Input: part model. Units: mm. Frame: model coordinates. A direction names the side the tool comes from. Round coordinates to 2 decimals unless told otherwise and drop trailing zeros. Loops run counter-clockwise (first coordinate to the right, second up) from the corner with the lowest first, then second, coordinate; pieces in that order, holes last. Notation, with made-up numbers: (38.25, 15) - (46.25, 15) arc R16 ccw to (46.25, 23) - close; hole circle Ø2 at (30.25, -35.75). An arc over 180 degrees is marked (long way). Write each question's results on one line, items separated by ' | '.
from build123d import *

# Parameters (mm, degrees)
BOSS_EXTRUDE1_DEPTH = 20
BOSS_EXTRUDE5_DEPTH = 5
SKETCH12_R          = 3
CUT_EXTRUDE7_DEPTH  = 88.776628115
SKETCH13_R          = 3
CUT_EXTRUDE8_DEPTH  = 87.566562518
SKETCH14_R          = 3
CUT_EXTRUDE9_DEPTH  = 91.441895398


with BuildPart() as part:
    # Sketch1 → Boss-Extrude1 (new body)
    with BuildSketch(Plane(origin=(0, 0, 0), x_dir=(1, 0, 0), z_dir=(0, 1, 0))):
        Polygon((0, 50), (0, 0), (40, 0), (40, 5), (5, 5), (5, 50), align=None)
    extrude(amount=BOSS_EXTRUDE1_DEPTH)

    # Sketch11 → Boss-Extrude5 (add)
    with BuildSketch(Plane(origin=(0, 20, 0), x_dir=(1, 0, 0), z_dir=(0, 1, 0))):
        Polygon((0, 0), (0, 15), (61.191009328, 48.995005183), (71.096669706, 31.164816504), (15, 0), align=None)
    extrude(amount=BOSS_EXTRUDE5_DEPTH)

    # Sketch12 → Cut-Extrude7 (cut, through all)
    with BuildSketch(Plane(origin=(0, 0, -5), x_dir=(-1, 0, 0), z_dir=(0, 0, -1))):
        with Locations((-10, 10)):
            Circle(SKETCH12_R)
        with Locations((-30, 10)):
            Circle(SKETCH12_R)
    extrude(amount=-CUT_EXTRUDE7_DEPTH, mode=Mode.SUBTRACT)

    # Sketch13 → Cut-Extrude8 (cut, through all)
    with BuildSketch(Plane(origin=(5, 0, 0), x_dir=(0, 0, -1), z_dir=(1, 0, 0))):
        with Locations((15, 10)):
            Circle(SKETCH13_R)
        with Locations((35, 10)):
            Circle(SKETCH13_R)
    extrude(amount=-CUT_EXTRUDE8_DEPTH, mode=Mode.SUBTRACT)

    # Sketch14 → Cut-Extrude9 (cut, through all)
    with BuildSketch(Plane(origin=(0, 25, 0), x_dir=(1, 0, 0), z_dir=(0, 1, 0))):
        with Locations(Location((57.323641314, 35.365007327, 0), (0, 0, 270))):
            Circle(SKETCH14_R)
        with Locations(Location((39.685556362, 25.936435896, 0), (0, 0, 270))):
            Circle(SKETCH14_R)
    extrude(amount=-CUT_EXTRUDE9_DEPTH, mode=Mode.SUBTRACT)


solid = part.part
1. Section query B-B, the plane y = 10. Output: boundary loops of the cut face in (x, z), plus the area to 3 significant figures.
Answer:
outline: (0, -50) - (5, -50) - (5, -38) - (0, -38) - close; (0, -32) - (5, -32) - (5, -18) - (0, -18) - close; (0, -12) - (5, -12) - (5, -5) - (7, -5) - (7, 0) - (0, 0) - close; (13, -5) - (27, -5) - (27, 0) - (13, 0) - close; (33, -5) - (40, -5) - (40, 0) - (33, 0) - close | area: 305 mm^2
2. Line query: line 1 (Y direction, x = 30, z = -2.2); line 2 (X direction, y = 3, z = -30.5); line 3 (Y direction, x = 2, z = -15). Output: solid intervals per line, ascending. Write a range as [from, to].
Answer:
line 1: [0, 7], [13, 20] | line 2: [0, 5] | line 3: [0, 7], [13, 25]
3. Section query D-D, the plane x = 10. Output: boundary loops of the cut face in (y, z), plus the area to 3 significant figures.
Answer:
outline: (0, -5) - (7, -5) - (7, 0) - (0, 0) - close; (13, -5) - (20, -5) - (20, -20.56) - (25, -20.56) - (25, 0) - (13, 0) - close | area: 173 mm^2
4. Section query A-A, the plane z = -30. Output: boundary loops of the cut face in (x, y), plus the area to 3 significant figures.
Answer:
outline: (0, 0) - (5, 0) - (5, 20) - (0, 20) - close; (27, 20) - (69, 20) - (69, 25) - (27, 25) - close | area: 310 mm^2
5. Contact query for flat-ended pins moving along their axis: pin 1 (4 mm diameter, centred on y = 5.5, z = -43.5, fed in from +X); pin 2 (2.5 mm diameter, centred on x = 1.5, z = -25, fed in from +Y); pin 3 (12 mm diameter, centred on x = 34, y = 22.5, fed in from +Z); pin 4 (12 mm diameter, centred on x = 59.5, y = 13, fed in from +Z). Output: stop coordinate, or through.
Answer:
pin 1: x = 5 | pin 2: y = 20 | pin 3: z = 0 | pin 4: through
6. Section query C-C, the plane z = -3. Output: boundary loops of the cut face in (x, y), plus the area to 3 significant figures.
Answer:
outline: (0, 0) - (40, 0) - (40, 20) - (20.4, 20) - (20.4, 25) - (0, 25) - close; hole circle Ø6 at (10, 10); hole circle Ø6 at (30, 10) | area: 845 mm^2
7. Mould query, pull axis Z, two halves, no side actions, for faces 1 (the flat face through (40, 10, -2)), 2 (the cylindrical face through (40.587, 22.535, -23.075)), 3 (the flat face through (30.17, 22.46, -31.76)), 4 (the cylindrical face through (2.5, 8.2, -12.6)). Classes: pulls with the +Z half, pulls with the -Z half, needs draft (parallel to the pull), parting line crosses it, or undercut.
Answer:
face 1: needs draft | face 2: undercut | face 3: pulls with the -Z half | face 4: undercut
8. Set-up query: faces 5 (the flat face through (30, 20, -3)), 6 (the flat face through (2, 20, -33)), 7 (the flat face through (39, 20, -22)). Return all of +Z, -Z, +X, -X, +Y, -Y with unobstructed straight access to the full face (end or side cutting, diameter ignored); none if empty.
Answer:
face 5: +Z, +X, +Y | face 6: -Z, -X, +Y | face 7: -Z, +X, -Y
